The listing builds one solid part. Answer for the finished solid, in the listing's coordinates (mm). A direction names the side the tool comes from. Give positions to 0.01 mm unless a question says otherwise; leave off trailing zeros. Write each loop counter-clockwise with the first axis right and the second up, starting at its lowest first coordinate (ties: lowest second). Pieces come first, ordered by that corner, then holes.
```python
from build123d import *

# Parameters (mm, degrees)
SKETCH_2_W               = 25
SKETCH_2_H               = 25
EXTRUDE_1_DEPTH          = 4
EXTRUDE_2_DEPTH          = 4
CUT_EXTRUDE_START        = -6
CUT_EXTRUDE_1_DEPTH      = 6
SKETCH_8_R               = 0.5
CUT_EXTRUDE_2_DEPTH      = 6
SKETCH_11_W              = 20.999639265
SKETCH_11_H              = 4
EXTRUDE_3_DEPTH          = 32
CUT_EXTRUDE_4_DEPTH      = 32
CUT_EXTRUDE_4_DEPTH_BACK = 32
SKETCH_13_R              = 1.25
SKETCH_13_W              = 12.5
SKETCH_13_H              = 22.7
CUT_EXTRUDE_5_DEPTH      = 41.264560711


with BuildPart() as part:
    # 草图2 → 凸台-拉伸1 (new body)
    with BuildSketch(Plane(origin=(0, 0, 0), x_dir=(1, 0, 0), z_dir=(0, 1, 0))):
        Rectangle(SKETCH_2_W, SKETCH_2_H)
    extrude(amount=EXTRUDE_1_DEPTH)

    # 草图3 → 凸台-拉伸2 (add)
    with BuildSketch(Plane(origin=(0, 4, 0), x_dir=(1, 0, 0), z_dir=(0, 1, 0))):
        with BuildLine():
            ThreePointArc((-3.5, 0), (-4.40433053, 2.347871376), (-6.65, 3.48245603))
            Line((-6.65, 3.48245603), (-6.65, -3.48245603))
            ThreePointArc((-6.65, -3.48245603), (-4.40433053, -2.347871376), (-3.5, 0))
        make_face()
        with BuildLine():
            Line((-6.65, -3.48245603), (-6.65, 3.48245603))
            ThreePointArc((-6.65, 3.48245603), (-10.5, 0), (-6.65, -3.48245603))
        make_face()
        with BuildLine():
            ThreePointArc((-3.5, 0), (-4.40433053, 2.347871376), (-6.65, 3.48245603))
            Line((-6.65, 3.48245603), (-6.65, -3.48245603))
            ThreePointArc((-6.65, -3.48245603), (-4.40433053, -2.347871376), (-3.5, 0))
        make_face()
        with BuildLine():
            Line((-6.65, -3.48245603), (-6.65, 3.48245603))
            ThreePointArc((-6.65, 3.48245603), (-10.5, 0), (-6.65, -3.48245603))
        make_face()
        with BuildLine():
            Line((8.2, 1.989974874), (-6.65, 3.48245603))
            ThreePointArc((-6.65, 3.48245603), (-4.40433053, 2.347871376), (-3.5, 0))
            ThreePointArc((-3.5, 0), (-4.40433053, -2.347871376), (-6.65, -3.48245603))
            Line((-6.65, -3.48245603), (8.2, -1.989974874))
            ThreePointArc((8.2, -1.989974874), (6, 0), (8.2, 1.989974874))
        make_face()
        with BuildLine():
            ThreePointArc((10, 0), (9.483239697, 1.341640786), (8.2, 1.989974874))
            Line((8.2, 1.989974874), (8.2, -1.989974874))
            ThreePointArc((8.2, -1.989974874), (9.483239697, -1.341640786), (10, 0))
        make_face()
        with BuildLine():
            Line((8.2, -1.989974874), (8.2, 1.989974874))
            ThreePointArc((8.2, 1.989974874), (6, 0), (8.2, -1.989974874))
        make_face()
        with BuildLine():
            ThreePointArc((10, 0), (9.483239697, 1.341640786), (8.2, 1.989974874))
            Line((8.2, 1.989974874), (8.2, -1.989974874))
            ThreePointArc((8.2, -1.989974874), (9.483239697, -1.341640786), (10, 0))
        make_face()
        with BuildLine():
            Line((8.2, -1.989974874), (8.2, 1.989974874))
            ThreePointArc((8.2, 1.989974874), (6, 0), (8.2, -1.989974874))
        make_face()
    extrude(amount=EXTRUDE_2_DEPTH)

    # 草图7 → 切除-拉伸1 (cut)
    with BuildSketch(Plane(origin=(0, 8, 0), x_dir=(1, 0, 0), z_dir=(0, 1, 0)).offset(CUT_EXTRUDE_START)):
        with BuildLine():
            Line((-6.65, -3.48245603), (8.2, -1.989974874))
            ThreePointArc((8.2, -1.989974874), (10, 0), (8.2, 1.989974874))
            Line((8.2, 1.989974874), (-6.65, 3.48245603))
            ThreePointArc((-6.65, 3.48245603), (-10.5, 0), (-6.65, -3.48245603))
        make_face()
    extrude(amount=CUT_EXTRUDE_1_DEPTH, mode=Mode.SUBTRACT)

    # 草图8 → 切除-拉伸2 (cut)
    with BuildSketch(Plane(origin=(0, 2, 0), x_dir=(1, 0, 0), z_dir=(0, 1, 0))):
        with Locations(Location((6, 0, 0), (0, 0, 270))):
            Circle(SKETCH_8_R)
    extrude(amount=-CUT_EXTRUDE_2_DEPTH, mode=Mode.SUBTRACT)

    # 草图11 → 凸台-拉伸3 (add)
    with BuildSketch(Plane.XZ):
        with Locations((2.000180367, 10.5)):
            Rectangle(SKETCH_11_W, SKETCH_11_H)
        Polygon((-8.499639265, 8.5), (-8.499639265, 12.5), (-12.5, 12.5), (-12.5, -12.5), (-8.499639265, -12.5), (-8.499639265, -8.5), align=None)
        with Locations((2.000180367, -10.5)):
            Rectangle(SKETCH_11_W, SKETCH_11_H)
    extrude(amount=EXTRUDE_3_DEPTH)

    # 草图12 → 切除-拉伸4 (cut, two sides: drawn at the far end of the back side and taken through both)
    with BuildSketch(Plane.XY.offset(-8.5).offset(-CUT_EXTRUDE_4_DEPTH_BACK)):
        Polygon((12.5, 0), (-8.499639265, -32), (12.5, -32), align=None)
    extrude(amount=CUT_EXTRUDE_4_DEPTH + CUT_EXTRUDE_4_DEPTH_BACK, mode=Mode.SUBTRACT)

    # 草图13 → 切除-拉伸5 (cut, through all)
    with BuildSketch(Plane(origin=(-8.499639265, 0, 0), x_dir=(0, 0, -1), z_dir=(1, 0, 0))):
        with Locations((0, -29.75)):
            Circle(SKETCH_13_R)
        with Locations((0, -2.25)):
            Circle(SKETCH_13_R)
        with Locations((0, -16)):
            Rectangle(SKETCH_13_W, SKETCH_13_H)
    extrude(amount=-CUT_EXTRUDE_5_DEPTH, mode=Mode.SUBTRACT)


solid = part.part
```
Item 1: A cutting plane is placed at B-B, the plane y = -11. Give the vertices of the cut face in (x, z), plus the area to 3 significant figures.
Conclusion:
outline: (-12.5, -12.5) - (5.28, -12.5) - (5.28, -8.5) - (-8.5, -8.5) - (-8.5, -6.25) - (-12.5, -6.25) - close; (-12.5, 6.25) - (-8.5, 6.25) - (-8.5, 8.5) - (5.28, 8.5) - (5.28, 12.5) - (-12.5, 12.5) - close
area: 160 mm2
Item 2: A cutting plane is placed at A-A, the plane z = 0. Give the vertices of the cut face in (x, y), plus the area to 3 significant figures.
Conclusion:
outline: (-12.5, -32) - (-8.5, -32) - (-8.5, -31) - (-12.5, -31) - close; (-12.5, -28.5) - (-8.5, -28.5) - (-8.5, -27.35) - (-12.5, -27.35) - close; (-12.5, -4.65) - (-8.5, -4.65) - (-8.5, -3.5) - (-12.5, -3.5) - close; (-12.5, -1) - (-8.5, -1) - (-8.5, 0) - (5.5, 0) - (5.5, 2) - (-10.5, 2) - (-10.5, 4) - (-12.5, 4) - close; (6.5, 0) - (12.5, 0) - (12.5, 4) - (10, 4) - (10, 2) - (6.5, 2) - close
area: 74.2 mm2
Item 3: A cutting plane is placed at C-C, the plane x = 6. Give the vertices of the cut face in (y, z).
Conclusion:
outline: (-9.9, -12.5) - (4, -12.5) - (4, -2.21) - (2, -2.21) - (2, -0.5) - (0, -0.5) - (0, -8.5) - (-9.9, -8.5) - close; (-9.9, 8.5) - (0, 8.5) - (0, 0.5) - (2, 0.5) - (2, 2.21) - (4, 2.21) - (4, 12.5) - (-9.9, 12.5) - close
Item 4: Each of these flat-tipped pins is pushed along its axis until it touches: P1, Ø4, axis at x = -7, z = 0, coming from the +Y side; P2, Ø1.5, axis at y = -29.75, z = 0, coming from the -X side; P3, Ø1.5, axis at x = 4, z = -8, coming from the -Y side; P4, Ø4, axis at y = -5, z = 1.5, coming from the +X side. Where does it stop, or does it pass through?
Conclusion:
P1: stops at y = 2
P2: passes through
P3: stops at y = -13.8
P4: stops at x = -8.5
Item 5: Consider probe 1 along Y at (x, z) = (-11.45, 0); probe 2 along Y at (x, z) = (-9.3, 0); probe 3 along Z at (x, y) = (-3.75, -9). Determine where each line is inside the solid, lowest interval first.
Conclusion:
probe 1: y = -32 to -31, -28.5 to -27.35, -4.65 to -3.5, -1 to 4
probe 2: y = -32 to -31, -28.5 to -27.35, -4.65 to -3.5, -1 to 2
probe 3: z = -12.5 to -8.5, 8.5 to 12.5
Item 6: Determine the mould class of faces 1 (the face through (-10, -4.65, 0)), 2 (the face through (-10.5, 3, -0.1)), 3 (the face through (2, -16, -11)) for opening direction X: pulls with the +X half, pulls with the -X half, needs draft (parallel to the pull), parting line crosses it, or undercut.
Conclusion:
face 1: needs draft
face 2: undercut
face 3: pulls with the +X half
Item 7: Which of the six approach directions +Z, -Z, +X, -X, +Y, -Y give full straight-line access (tool end or side, diameter ignored) to faces 4 (the face through (-10, -16, 6.25)), 5 (the face through (0.879, 2.986, -2.726)), 6 (the face through (0, -12, -8.5))?
Conclusion:
face 4: +X, -X
face 5: +Y
face 6: +X, -Y
Item 8: A cutting plane is placed at D-D, the plane z = 10. Give the vertices of the cut face in (x, y), plus the area to 3 significant figures.
Conclusion:
outline: (-12.5, -32) - (-8.5, -32) - (12.5, 0) - (12.5, 4) - (-12.5, 4) - close
area: 564 mm2
